Drawing for the job (mm, zero at the part's lowest x, y, z). Coordinates: 2 decimals unless noted, no trailing zeros. Order: outer loops, then holes, each group sorted by start corner. A loop starts at its lowest first (then second) coordinate and runs counter-clockwise, first axis right, second up. Notation, with made-up numbers: (3.25, 41.5) - (55.25, 41.5) arc R16 cw to (55.25, 60.5) - close; hole circle Ø10 at (20, 24.25). An arc over 180 degrees is marked (long way). Put each result on its own line as item: value. Start each with the question number.
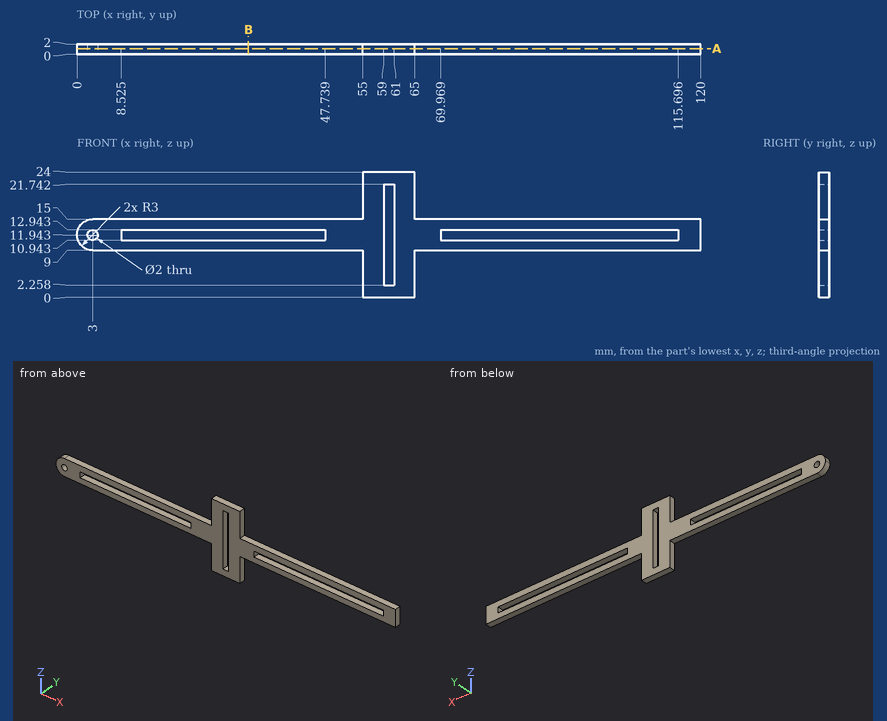
Item 1: Flat gauge pins, fed straight in: pin 1 Ø1 at (x, y) = (76.5, 1) entering from -Z; pin 2 Ø1 at (x, y) = (95, 1.5) entering from +Z; pin 3 Ø6 at (x, z) = (45.5, 5.5) entering from -Y; pin 4 Ø1 at (y, z) = (1, 4) entering from +X. Where does each tip first touch, or does it go through?
Item 2: Slice it at B-B, the plane x = 33. Give the cut face in (y, z).
Item 3: Slice it at A-A, the plane y = 1.1. Give the number of separate pieces and of enclosed holes in the cut face.
Item 4: Wall check: line 1 along Z through (x, y) = (113.5, 1.7); line 2 along X through (y, z) = (0.6, 16.25); line 3 along X through (y, z) = (1.65, 11.5) (1 decimal). Give the ranges that are in metal, low to high.
Here are the results:
1. pin 1: stops at z = 9
1. pin 2: stops at z = 15
1. pin 3: passes through
1. pin 4: stops at x = 65
2. outline: (0, 9) - (2, 9) - (2, 10.94) - (0, 10.94) - close; (0, 12.94) - (2, 12.94) - (2, 15) - (0, 15) - close
3. separate pieces: 1
3. enclosed holes: 4
4. line 1: z = 9 to 10.94, 12.94 to 15
4. line 2: x = 55 to 59, 61 to 65
4. line 3: x = 0 to 2.1, 3.9 to 8.5, 47.7 to 59, 61 to 70, 115.7 to 120
